Check sheet for the modelled part. Datum: model origin and axes. Units: mm. A direction names the side the tool comes from. Round coordinates to 2 decimals unless told otherwise and drop trailing zeros. Loops run counter-clockwise (first coordinate to the right, second up) from the corner with the lowest first, then second, coordinate; pieces in that order, holes last. Notation, with made-up numbers: (43, -3.5) - (74, -3.5) arc R25 cw to (74, 16.5) - close; hole circle Ø7 at (84.25, 52). An arc over 180 degrees is marked (long way). Answer in a Markdown table with one row per item. Add a question column.
(1) Cross-section at C-C on y = 0. Enter the section's corners in (x, z).
(2) Cross-section at A-A on x = 0.8. Enter the section's corners in (y, z), then the cut area to 3 significant figures.
(3) Gauge pin test, flat end, axial feed: pin 1 (3 mm diameter, centred on y = 19, z = 0, fed in from -X). Record the tip position at first contact, or that the pin passes through.
(4) Access from +Z, -Z, +X, -X, +Y, -Y to the whole of each face (thin tool, end or side, straight path). Record for faces 4 (the flat face through (1, -2.75, 0)), 5 (the flat face through (0.74, 13.4, -8.11)).
(5) Cross-section at B-B on z = -3. Enter the section's corners in (x, y), then the cut area to 3 significant figures.
(6) Mould release check, pull along Y, two halves, no side actions. Record for faces 1 (the flat face through (0.74, 13.18, 8.214)), 2 (the cylindrical face through (1, -13, 0)), 3 (the flat face through (0.74, 1.317, 2.415)): +Y half, -Y half, draft (parallel to the pull), parting line (faces both ways), or undercut.
(7) Cross-section at D-D on z = 8.25. Enter the section's corners in (x, y).
(8) Thickness scan on line 1 along Y through (x, z) = (1.05, 1); line 2 along Z through (x, y) = (1.35, 4); line 3 along Z through (x, y) = (1.25, 17). Record the ranges inside material, lowest first.
from build123d import *

# Parameters (mm, degrees)
SKETCH1_R           = 2.5
BOSS_EXTRUDE1_DEPTH = 1.5


with BuildPart() as part:
    # Sketch1 → Boss-Extrude1 (new body)
    with BuildSketch(Plane(origin=(0, 0, 0), x_dir=(0, 0, -1), z_dir=(1, 0, 0))):
        with BuildLine():
            Line((-11.791470696, 5.473684211), (-4.535181037, 21.105263158))
            ThreePointArc((-4.535181037, 21.105263158), (0, 24), (4.535181037, 21.105263158))
            Line((4.535181037, 21.105263158), (11.791470696, 5.473684211))
            ThreePointArc((11.791470696, 5.473684211), (0, -13), (-11.791470696, 5.473684211))
        make_face()
        with Locations((0, 19)):
            Circle(SKETCH1_R, mode=Mode.SUBTRACT)
        Polygon((4.763139721, -2.75), (-4.763139721, -2.75), (0, 5.5), align=None, mode=Mode.SUBTRACT)
    extrude(amount=BOSS_EXTRUDE1_DEPTH)


solid = part.part
Answers:
| question | item | result |
|---|---|---|
| 1 | outline | (0, -13) - (1.5, -13) - (1.5, -3.18) - (0, -3.18) - close; (0, 3.18) - (1.5, 3.18) - (1.5, 13) - (0, 13) - close |
| 2 | outline | (5.47, -11.79) - (21.11, -4.54) arc R5 ccw to (21.11, 4.54) - (5.47, 11.79) arc R13 ccw (long way) to start; hole (-2.75, -4.76) - (5.5, 0) - (-2.75, 4.76) - close; hole circle Ø5 at (19, 0) |
| 2 | area | 619 mm^2 |
| 3 | pin 1 | passes through |
| 4 | face 4 | +X, -X |
| 4 | face 5 | -Z, +X, -X, +Y |
| 5 | outline | (0, -12.65) - (1.5, -12.65) - (1.5, -2.75) - (0, -2.75) - close; (0, 0.3) - (1.5, 0.3) - (1.5, 23) - (0, 23) - close |
| 5 | area | 48.9 mm^2 |
| 6 | face 1 | +Y half |
| 6 | face 2 | parting line |
| 6 | face 3 | undercut |
| 7 | outline | (0, -10.05) - (1.5, -10.05) - (1.5, 13.1) - (0, 13.1) - close |
| 8 | line 1 | y = -12.96 to -2.75, 3.77 to 16.71, 21.29 to 23.9 |
| 8 | line 2 | z = -12.37 to -0.87, 0.87 to 12.37 |
| 8 | line 3 | z = -6.44 to -1.5, 1.5 to 6.44 |
